Check sheet for the drawn part. Datum: minimum x, y, z corner. Units: mm. A direction names the side the tool comes from. Round coordinates to 2 decimals unless told otherwise and drop trailing zeros. Order: outer loops, then holes, each group sorted by start corner. A loop starts at its lowest first (then second) coordinate and runs counter-clockwise, first axis right, second up. Notation, with made-up numbers: (14.25, 33) - (70.25, 33) arc R27 ccw to (70.25, 69) - close; hole circle Ø3 at (88, 67.25). An arc over 180 degrees is marked (long way). Write each question's results on one line, items separated by ' | '.
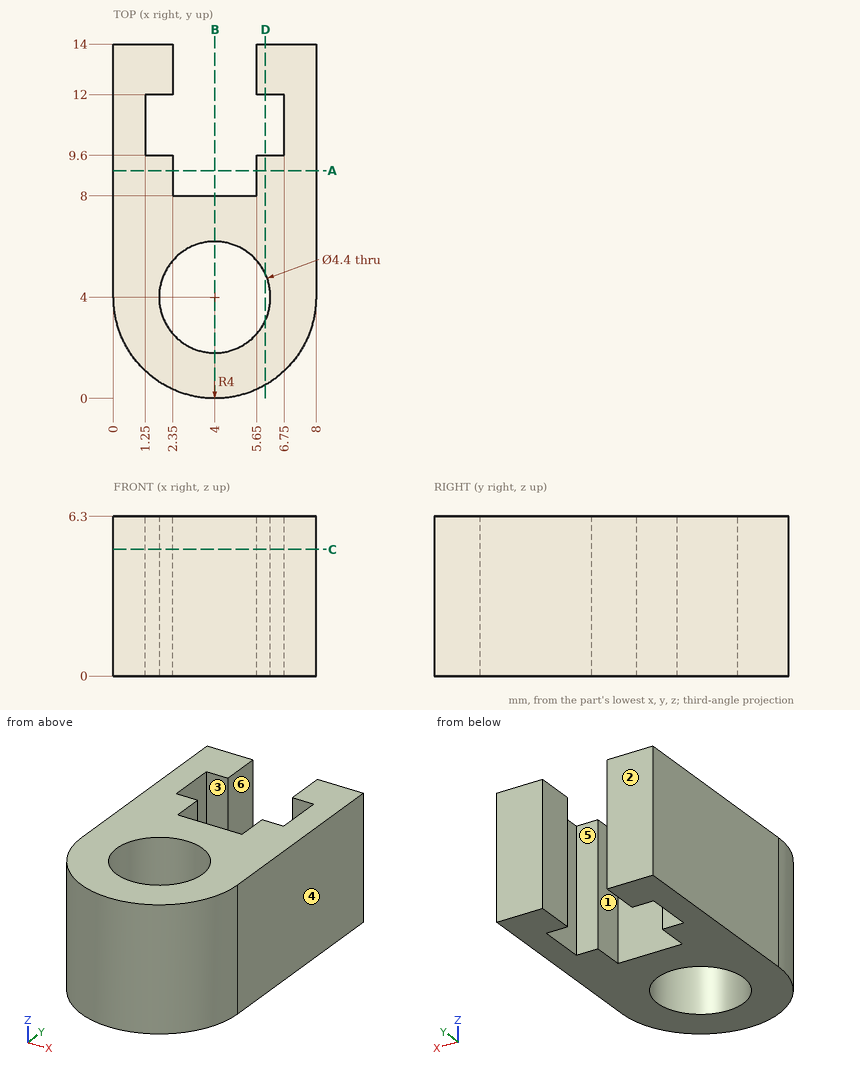
(1) Section check A-A (y = 9). Record the cut outline in (x, z), then the cut area to 3 significant figures.
Answers follow:
outline: (0, 0) - (2.35, 0) - (2.35, 6.3) - (0, 6.3) - close; (5.65, 0) - (8, 0) - (8, 6.3) - (5.65, 6.3) - close | area: 29.6 mm²
(2) Section check D-D (x = 6). Record the cut outline in (y, z), then the cut area to 3 significant figures.
Answers follow:
outline: (0.54, 0) - (3.08, 0) - (3.08, 6.3) - (0.54, 6.3) - close; (4.92, 0) - (9.6, 0) - (9.6, 6.3) - (4.92, 6.3) - close; (12, 0) - (14, 0) - (14, 6.3) - (12, 6.3) - close | area: 58.2 mm²
(3) Section check C-C (z = 5). Record the cut outline in (x, y), then the cut area to 3 significant figures.
Answers follow:
outline: (0, 4) arc R4 ccw to (8, 4) - (8, 14) - (5.65, 14) - (5.65, 12) - (6.75, 12) - (6.75, 9.6) - (5.65, 9.6) - (5.65, 8) - (2.35, 8) - (2.35, 9.6) - (1.25, 9.6) - (1.25, 12) - (2.35, 12) - (2.35, 14) - (0, 14) - close; hole circle Ø4.4 at (4, 4) | area: 64.8 mm²
(4) Material ranges on line 1 (Y direction, x = 4, z = 4); line 2 (X direction, y = 8.5, z = 4.75); line 3 (X direction, y = 11.5, z = 4.75), recorded low to high.
Answers follow:
line 1: 0 to 1.8, 6.2 to 8 | line 2: 0 to 2.35, 5.65 to 8 | line 3: 0 to 1.25, 6.75 to 8
(5) Depth check by flat-ended pin: pin 1 Ø1.8 at (y, z) = (9, 3) entering from -X; pin 2 Ø2.5 at (x, z) = (4, 3) entering from +Y; pin 3 Ø0.9 at (x, z) = (2, 3) entering from -Y. Enter the tip coordinate at first touch or a pass-through.
Answers follow:
pin 1: x = 0 | pin 2: y = 8 | pin 3: y = 0.31
(6) Draft check along Y on the marked faces 1, 2 and 3. Enter one of: released by +Y, released by -Y, zero draft, split by the parting line, or undercut.
Answers follow:
face 1: zero draft | face 2: released by +Y | face 3: undercut
(7) Section check B-B (x = 4). Record the cut outline in (y, z).
Answers follow:
outline: (0, 0) - (1.8, 0) - (1.8, 6.3) - (0, 6.3) - close; (6.2, 0) - (8, 0) - (8, 6.3) - (6.2, 6.3) - close
(8) Access from +Z, -Z, +X, -X, +Y, -Y to the whole of each face (thin tool, end or side, straight path). Record for the marked faces 4, 5 and 6.
Answers follow:
face 4: +Z, -Z, +X, +Y, -Y | face 5: +Z, -Z | face 6: +Z, -Z, +Y
